Part print with two shaded views. Sizes in mm from the minimum x, y, z corner. A direction names the side the tool comes from. Coordinates: 2 decimals unless noted, no trailing zeros. Write each loop counter-clockwise with the first axis right and the second up, starting at its lowest first coordinate (ties: lowest second). Pieces come first, ordered by that corner, then holes. Notation, with made-up numbers: (75.5, 60) - (106.5, 60) arc R25 cw to (106.5, 89) - close; hole circle Ø11 at (-38.75, 51). An arc over 180 degrees is marked (long way). Answer in a Markdown table with one row per item. Add a question column.
Q1. Band-saw the part on C-C (y = 2.25). List the corners of the cut face in (x, z) (1 decimal), and give its area (3 significant figures).
Q2. Band-saw the part on B-B (x = 2.1). List the corners of the cut face in (y, z).
Q3. 3-axis set-ups, long thin cutter, end or side, ignore diameter. For the marked faces 1, 2 and 3: which of +Z, -Z, +X, -X, +Y, -Y reach the whole face in a straight line?
Q4. Band-saw the part on D-D (y = 8.75). List the corners of the cut face in (x, z).
Q5. Band-saw the part on A-A (z = 1.45). List the corners of the cut face in (x, y) (1 decimal).
Q6. Drill centre lines: line 1 along Y through (x, z) = (1.7, 2.45); line 2 along Y through (x, z) = (4.05, 1.35); line 3 along Z through (x, y) = (2.5, 1). Where is each one in solid material? Low to high. Write a range as from..to.
Q7. Pin check, flat tips, straight feed: pin 1 (1 mm diameter, centred on x = 1.5, y = 6, fed in from -Z); pin 2 (0.6 mm diameter, centred on x = 2.5, z = 1.5, fed in from -Y). Stop position of each tip, or through.
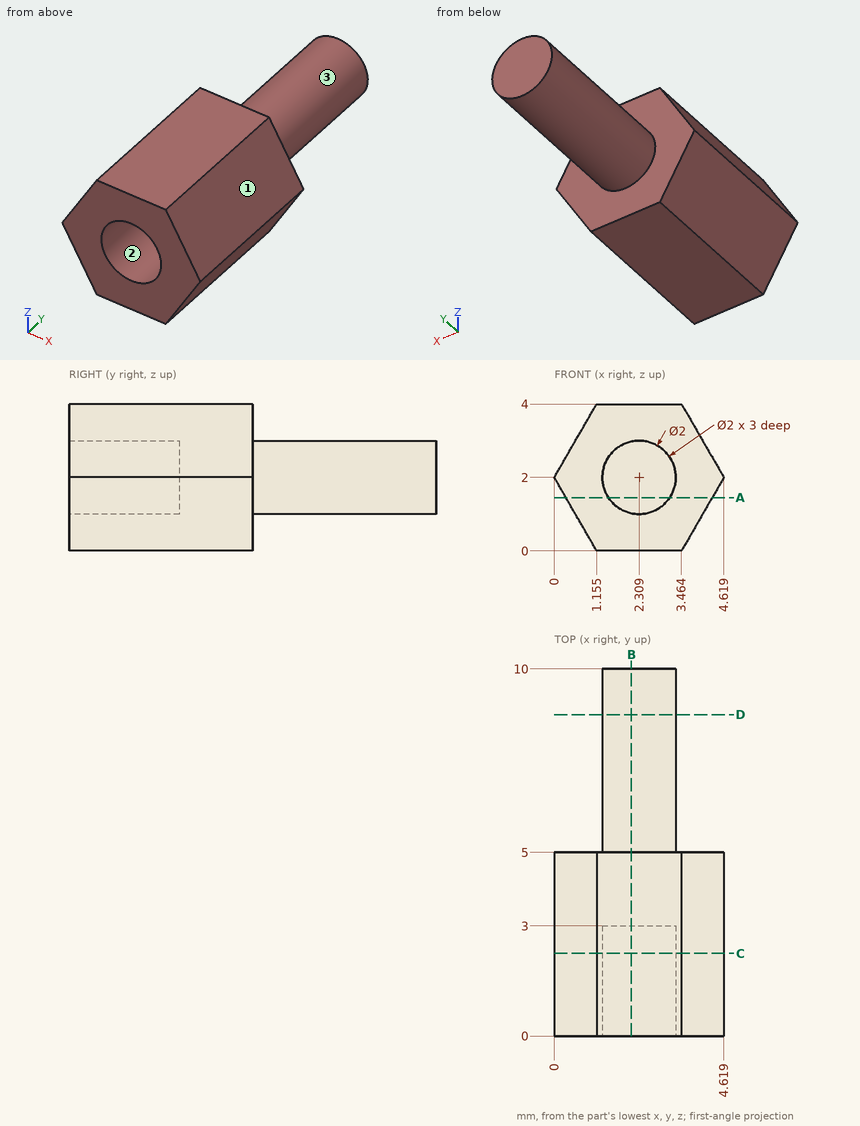
Checked values:
| question | item | result |
|---|---|---|
| 1 | outline | (0, 2) - (1.2, 0) - (3.5, 0) - (4.6, 2) - (3.5, 4) - (1.2, 4) - close; hole circle Ø2 at (2.3, 2) |
| 1 | area | 10.7 mm² |
| 2 | outline | (0, 0) - (5, 0) - (5, 1.02) - (10, 1.02) - (10, 2.98) - (5, 2.98) - (5, 4) - (0, 4) - (0, 2.98) - (3, 2.98) - (3, 1.02) - (0, 1.02) - close |
| 3 | face 1 | +Z, +X, +Y, -Y |
| 3 | face 2 | -Y |
| 3 | face 3 | +Y |
| 4 | outline | circle Ø2 at (2.31, 2) |
| 5 | outline | (0.3, 0) - (1.5, 0) - (1.5, 3) - (3.1, 3) - (3.1, 0) - (4.3, 0) - (4.3, 5) - (3.1, 5) - (3.1, 10) - (1.5, 10) - (1.5, 5) - (0.3, 5) - close |
| 6 | line 1 | y = 3..10 |
| 6 | line 2 | y = 0..5 |
| 6 | line 3 | z = 0..1.02, 2.98..4 |
| 7 | pin 1 | stops at z = 1.05 |
| 7 | pin 2 | stops at y = 3 |
